Input: part model. Units: mm. Frame: model coordinates. Give positions to 0.01 mm unless a question says otherwise; leave off trailing zeros. Loops run counter-clockwise (first coordinate to the right, second up) from the corner with the lowest first, then second, coordinate; pieces in that order, holes last. Notation, with made-up numbers: (33, 89) -> (47, 89) arc R5 cw to (47, 96) -> close; hole circle Ø5 at (-1, -27.5). An arc over 180 degrees is marked (long way). Answer as a JSON object with one key per item and string values. Group by question number.
Autodesk Inventor part; units mm, degrees
ref_plane "YZ Plane" through (0, 0, 0) normal (1, 0, 0) x (0, 1, 0)
ref_plane "XZ Plane" through (0, 0, 0) normal (0, 1, 0) x (-1, 0, 0)
ref_plane "XY Plane" through (0, 0, 0) normal (0, 0, 1) x (1, 0, 0)
sketch "Sketch2" plane through (0, 0, 0) normal (0, 0, 1) x (1, 0, 0)
  circle A0 centre (0, 0) radius 37.5031
  dimension "d0" = 75.0062
extrude "Extrusion1" add sketch "Sketch2" against normal blind 3.048
sketch "Sketch3" plane through (0, 0, -3.048) normal (0, 0, -1) x (-1, 0, 0)
  circle A0 centre (0, 0) radius 37.5031
extrude "Extrusion2" add sketch "Sketch3" along normal blind 2.032 draft -75
sketch "Sketch4" plane through (0, 0, 0) normal (0, 0, 1) x (1, 0, 0)
  circle A0 centre (0, 0) radius 37.5031
  circle A1 centre (0, 0) radius 26.0985
  dimension "d5" = 52.197
extrude "Extrusion3" cut sketch "Sketch4" against normal blind 2.54 contours A1
sketch "Sketch5" plane through (0, 0, -5.08) normal (0, 0, -1) x (-1, 0, 0)
  circle A0 centre (0, 0) radius 29.9196
hole "Hole1" at (0, 0, -5.08) direction (0, 0, 1) diameter 49.2252 end through all counterbore diameter 51.054 counterbore depth 1.27
properties part number "4000120" material "304L Stainless Steel"
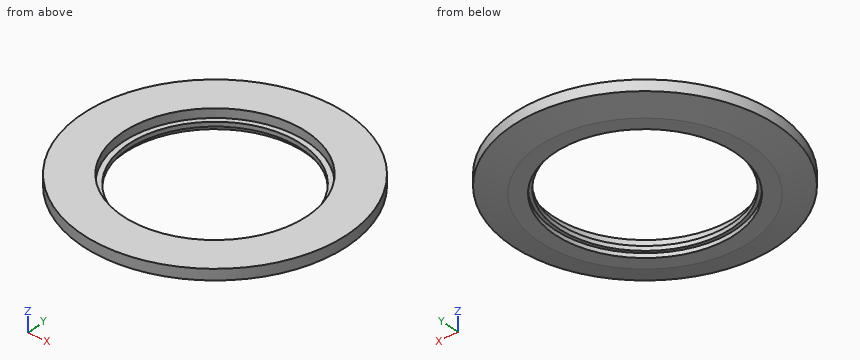
Q1. Pin query (flat end, axial travel): pin 1 Ø3 at (x, z) = (-7.5, -2.5) entering from -Y; pin 2 Ø3 at (y, z) = (-23, -1.5) entering from -X; pin 3 Ø3 at (y, z) = (-7.5, -1) entering from -X; pin 4 Ø10 at (x, y) = (-14, 8) entering from -Z. Return the tip coordinate at first contact, or that it passes through.
Q2. Section A-A on x = 0. Return the cut outline in (y, z), then the cut area to 3 significant figures.
Q3. Section B-B on z = -0.9. Return the cut outline in (x, y), then the cut area to 3 significant figures.
Q4. Ray query, probe 1 along Y at (x, z) = (0, -2.9); probe 2 along X at (y, z) = (-19.5, -0.4); probe 3 along Y at (x, z) = (-17.5, -1.7). Return the intervals inside material, ascending.
Numbers:
{
 "1": {"pin 1": "stops at y = -37.02", "pin 2": "stops at x = -30.73", "pin 3": "stops at x = -37.02", "pin 4": "passes through"},
 "2": {"outline": "(-37.5, -3.05) -> (-29.92, -5.08) -> (-25.53, -5.08) -> (-25.53, -3.81) -> (-24.61, -3.81) -> (-24.61, -2.54) -> (-26.1, -2.54) -> (-26.1, 0) -> (-37.5, 0) -> close; (24.61, -3.81) -> (25.53, -3.81) -> (25.53, -5.08) -> (29.92, -5.08) -> (37.5, -3.05) -> (37.5, 0) -> (26.1, 0) -> (26.1, -2.54) -> (24.61, -2.54) -> close", "area": "106 mm²"},
 "3": {"outline": "circle Ø75.01 at (0, 0); hole circle Ø52.2 at (0, 0)", "area": "2,280 mm²"},
 "4": {"probe 1": "y = -37.5 to -24.61, 24.61 to 37.5", "probe 2": "x = -32.03 to -17.35, 17.35 to 32.03", "probe 3": "y = -33.17 to -19.36, 19.36 to 33.17"}
}
